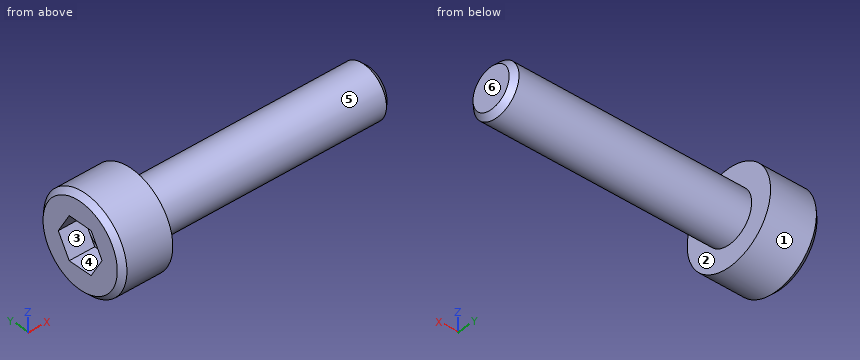
Autodesk Inventor part; units mm, degrees
ref_plane "to_cp_XY" through (0, 0, 0) normal (1, 0, 0) x (0, 0, -1)
ref_plane "to_cp_YZ" through (0, 0, 0) normal (0, 0, -1) x (0, 1, 0)
ref_plane "to_cp_ZX" through (0, 0, 0) normal (0, 1, 0) x (1, 0, 0)
sketch "Sketch_1" plane through (0, 0, 0) normal (0, 0, 1) x (1, 0, 0)
  line L0 (14, 0) -> (-3, 0)
  line L1 (-3, 0) -> (-3, 2.45)
  line L2 (-3, 2.45) -> (-2.7, 2.75)
  line L3 (-2.7, 2.75) -> (0, 2.75)
  line L4 (0, 2.75) -> (0, 1.5)
  line L5 (0, 1.5) -> (13.6935, 1.5)
  line L6 (13.6935, 1.5) -> (14, 1.1935)
  line L7 (14, 1.1935) -> (14, 0)
  line L8 (14, 0) -> (-3, 0)
revolve "Revolution1" add sketch "Sketch_1" angle 360 about axis through (14, 0, 0) along (1, 0, 0)
thread "Thread1"
sketch "Sketch2" plane through (-3, 0, 0) normal (-1, 0, 0) x (0, 0, 1)
  point P0 (0, 0)
hole "Hole1" at (-3, 0, 0) direction (1, 0, 0) diameter 2.5 depth 1.5 tip angle 150
sketch "Sketch_3" plane through (-3, 0, 0) normal (1, 0, 0) x (0, 0, -1)
  line L0 (-1.25, -0.7217) -> (0, -1.4434)
  line L1 (0, -1.4434) -> (1.25, -0.7217)
  line L2 (1.25, -0.7217) -> (1.25, 0.7217)
  line L3 (1.25, 0.7217) -> (0, 1.4434)
  line L4 (0, 1.4434) -> (-1.25, 0.7217)
  line L5 (-1.25, 0.7217) -> (-1.25, -0.7217)
extrude "Extrusion1" cut sketch "Sketch_3" along normal blind 1.5
ref_plane "to_cp_XY" through (0, 0, 0) normal (1, 0, 0) x (0, 0, -1)
ref_plane "to_cp_YZ" through (0, 0, 0) normal (0, 0, -1) x (0, 1, 0)
ref_plane "to_cp_ZX" through (0, 0, 0) normal (0, 1, 0) x (1, 0, 0)
properties part number "BOLT3-14"
Here's how the part is built. I have some questions about the finished solid (model axes, mm). Face numbers are marked on the shaded views. A direction names the side the tool comes from. Round coordinates to 2 decimals unless told otherwise and drop trailing zeros. Write each loop counter-clockwise with the first axis right and the second up, starting at its lowest first coordinate (ties: lowest second). Pieces come first, ordered by that corner, then holes.
1. Suppose I cut it at A-A (x = -0.5). List the corners of the cut face in (y, z) for me.
2. If we mould it in two halves opening along Z, with no side actions, what happens to the marked faces 4, 5 and 6? For each: released by +Z, released by -Z, zero draft, split by the parting line, or undercut.
3. I need wall thicknesses on L1, parallel to X at y = -0.1, z = 1.85; L2, parallel to Y at x = 6, z = -0.4; L3, parallel to Z at x = 6.5, y = 0. Which ranges of each line are inside material? Lowest first, please.
4. Will this pin go through, and if not, where does the flat tip stop? pin 1 Ø1 at (x, z) = (6, -0.5) entering from +Y.
5. Suppose I cut it at B-B (x = 3). List the corners of the cut face in (y, z) for me, and give its area (3 significant figures).
6. For the marked faces 1, 2 and 3, which set-ups out of +Z, -Z, +X, -X, +Y, -Y let a thin tool reach every point of the face, with its end or its side?
Answer sheet:
1. outline: circle Ø5.5 at (0, 0)
2. face 4: undercut
2. face 5: split by the parting line
2. face 6: zero draft
3. L1: x = -3 to 0
3. L2: y = -1.45 to 1.45
3. L3: z = -1.5 to 1.5
4. pin 1: stops at y = 1.5
5. outline: circle Ø3 at (0, 0)
5. area: 7.07 mm2
6. face 1: +X, -X
6. face 2: +X
6. face 3: -X
